from build123d import *

# Parameters (mm, degrees)
SKETCH1_R           = 14.3002
BOSS_EXTRUDE1_DEPTH = 6.35
FILLET1_R           = 10.16


with BuildPart() as part:
    # Sketch1 → Boss-Extrude1 (new body)
    with BuildSketch(Plane.XY):
        with BuildLine():
            Line((-54.787568662, -25.4), (0, -25.4))
            ThreePointArc((0, -25.4), (22.465756024, 11.851152107), (-20.96418046, 14.340960136))
            ThreePointArc((-20.96418046, 14.340960136), (-96.891931571, 296.382201918), (193.491662983, 327.840960136))
            ThreePointArc((193.491662983, 327.840960136), (200.114883307, 292.53581954), (235.420023903, 299.159039864))
            ThreePointArc((235.420023903, 299.159039864), (259.695607277, 301.436411104), (261.893582664, 325.719311922))
            ThreePointArc((261.893582664, 325.719311922), (14.357413322, 426.207029502), (-175.89272439, 238.652179878))
            Line((-175.89272439, 238.652179878), (-226.69272439, 238.652179878))
            Line((-226.69272439, 238.652179878), (-226.69272439, 137.052179878))
            Line((-226.69272439, 137.052179878), (-175.89272439, 137.052179878))
            ThreePointArc((-175.89272439, 137.052179878), (-133.078613493, 42.602384317), (-54.787568662, -25.4))
        make_face()
        Circle(SKETCH1_R, mode=Mode.SUBTRACT)
        with Locations((214.455843443, 313.5)):
            Circle(SKETCH1_R, mode=Mode.SUBTRACT)
    extrude(amount=BOSS_EXTRUDE1_DEPTH)

    # Fillet1
    fillet1_edges = [part.edges().sort_by_distance(p)[0] for p in [
        (-54.787568662, -25.4, 3.175),
        (-175.89272439, 137.052179878, 3.175),
        (-175.89272439, 238.652179878, 3.175),
    ]]
    fillet(fillet1_edges, radius=FILLET1_R)


solid = part.part
Check sheet for the modelled part. Datum: model origin and axes. Units: mm. Give positions to 0.01 mm unless a question says otherwise; leave off trailing zeros. Loops run counter-clockwise (first coordinate to the right, second up) from the corner with the lowest first, then second, coordinate; pieces in that order, holes last. Notation, with made-up numbers: M 4.25,-30 L 41.25,-30 A21 ccw 41.25,9 Z; hole C -33.5,59 d2. An arc over 180 degrees is marked long. Return JSON: item names as keys, results as strings. Group by question number.
1. Cross-section at D-D on x = 177. Record the boundary of the cut face in (y, z).
2. Go/stop test with flat-tipped pins: pin 1 (1.5 mm diameter, centred on x = -59.5, z = 2, fed in from +Y); pin 2 (1.9 mm diameter, centred on x = -205, z = 3, fed in from -Y); pin 3 (1 mm diameter, centred on x = 23.5, z = 2.5, fed in from -Y). Record where each tip stops, or that it passes through.
3. Cross-section at C-C on y = 0. Record the boundary of the cut face in (x, z).
4. Cross-section at A-A on y = 313.5. Record the boundary of the cut face in (x, z), plus the area to 3 significant figures.
5. Thickness scan on L1, parallel to X at y = 305, z = 1.5; L2, parallel to Y at x = 66.5, z = 6.25; L3, parallel to X at y = 6, z = 6. Record the ranges inside material, lowest first.
6. Mould release check, pull along X, two halves, no side actions. Record for faces 1 (the flat face through (-91, 305, 0)), 2 (the cylindrical face through (-132.34, 41.62, 3.13)), 3 (the cylindrical face through (259.432, 301.177, 3.131)), 4 (the cylindrical face through (22.093, 427.616, 3.131)): released by +X, released by -X, zero draft, split by the parting line, or undercut.
7. Cross-section at B-B on z = 3. Record the boundary of the cut face in (x, y), plus the area to 3 significant figures.
Return value:
{
 "1": {"outline": "M 341.7,0 L 401.82,0 L 401.82,6.35 L 341.7,6.35 Z"},
 "2": {"pin 1": "y = 398.89", "pin 2": "y = 137.05", "pin 3": "y = -10.78"},
 "3": {"outline": "M -92.42,0 L -14.3,0 L -14.3,6.35 L -92.42,6.35 Z; M 14.3,0 L 25.4,0 L 25.4,6.35 L 14.3,6.35 Z"},
 "4": {"outline": "M -146.26,0 L -83.71,0 L -83.71,6.35 L -146.26,6.35 Z; M 189.06,0 L 200.16,0 L 200.16,6.35 L 189.06,6.35 Z; M 228.76,0 L 265.21,0 L 265.21,6.35 L 228.76,6.35 Z", "area": "699 mm^2"},
 "5": {"L1": "-151.16 to -90.64, 190.52 to 202.96, 225.96 to 262.49", "L2": "380.02 to 430.83", "L3": "-99.45 to -12.98, 12.98 to 24.68"},
 "6": {"face 1": "zero draft", "face 2": "released by -X", "face 3": "undercut", "face 4": "split by the parting line"},
 "7": {"outline": "M -226.69,137.05 L -183.97,137.05 A10.16 cw -174.11,129.34 A243.02 ccw -57.13,-24.1 A10.16 ccw -52.16,-25.4 L 0,-25.4 A25.4 ccw long -20.96,14.34 A192.22 cw long 193.49,327.84 A25.4 ccw 235.42,299.16 A19.07 ccw 261.89,325.72 A243.02 ccw -174.11,246.37 A10.16 cw -183.97,238.65 L -226.69,238.65 Z; hole C 0,0 d28.6; hole C 214.46,313.5 d28.6", "area": "47,800 mm^2"}
}
